Check sheet for the modelled part. Datum: model origin and axes. Units: mm. A direction names the side the tool comes from. Round coordinates to 2 decimals unless told otherwise and drop trailing zeros. Write each loop counter-clockwise with the first axis right and the second up, starting at its lowest first coordinate (ties: lowest second). Pieces come first, ordered by that corner, then holes. Notation, with made-up numbers: M -25.75,79.5 L -7.75,79.5 A26 cw -7.75,97.5 Z; hole C -14.5,66.5 d7. An arc over 180 degrees is marked long. Answer in a Markdown table with one row per item.
```python
from build123d import *

# Parameters (mm, degrees)
SKETCH_1_R       = 1.6
EXTRUDE_1_DEPTH  = 2
CHAMFER_1_SIZE   = 5
FILLET_START     = -1
FILLET_1_DEPTH   = 4
FILLET_1_2_DEPTH = 2
FILLET_2_R       = 3


with BuildPart() as part:
    # 草图1 → 凸台-拉伸1 (new body)
    with BuildSketch(Plane(origin=(0, 0, 0), x_dir=(1, 0, 0), z_dir=(0, 1, 0))):
        Polygon((-10, -14), (-10, 14), (10, 14), (10, 6), (30, 6), (30, -6), (10, -6), (10, -14), align=None)
        with Locations(Location((0, 10, 0), (0, 0, 270))):
            Circle(SKETCH_1_R, mode=Mode.SUBTRACT)
        with Locations(Location((0, -10, 0), (0, 0, 90))):
            Circle(SKETCH_1_R, mode=Mode.SUBTRACT)
        with Locations(Location((17.5, 0, 0), (0, 0, 270))):
            Circle(SKETCH_1_R, mode=Mode.SUBTRACT)
        with Locations(Location((24.5, 0, 0), (0, 0, 270))):
            Circle(SKETCH_1_R, mode=Mode.SUBTRACT)
    extrude(amount=EXTRUDE_1_DEPTH)

    # 倒角1
    chamfer_1_edges = [part.edges().sort_by_distance(p)[0] for p in [
        (10, 1, 14),
        (-10, 1, 14),
        (-10, 1, -14),
        (10, 1, -14),
    ]]
    chamfer(chamfer_1_edges, length=CHAMFER_1_SIZE)

    # 圆角1: read off the stored shape, not the designer's step
    # 圆角1 outline → 圆角1 (cut)
    with BuildSketch(Plane(origin=(0, 0, 0), x_dir=(1, 0, 0), z_dir=(0, 1, 0)).offset(FILLET_START)):
        with BuildLine():
            ThreePointArc((27, 6), (29.121320344, 5.121320344), (30, 3))
            Line((30, 3), (30, 6))
            Line((30, 6), (27, 6))
        make_face()
        with BuildLine():
            ThreePointArc((30, -3), (29.121320344, -5.121320344), (27, -6))
            Line((27, -6), (30, -6))
            Line((30, -6), (30, -3))
        make_face()
    extrude(amount=FILLET_1_DEPTH, mode=Mode.SUBTRACT)

    # Fillet 1 2 outline → Fillet 1 2 (add)
    with BuildSketch(Plane(origin=(0, 0, 0), x_dir=(1, 0, 0), z_dir=(0, 1, 0))):
        with BuildLine():
            Line((10, 6), (13, 6))
            ThreePointArc((13, 6), (10.878679656, 6.878679656), (10, 9))
            Line((10, 9), (10, 6))
        make_face()
        with BuildLine():
            ThreePointArc((10, -9), (10.878679656, -6.878679656), (13, -6))
            Line((13, -6), (10, -6))
            Line((10, -6), (10, -9))
        make_face()
    extrude(amount=FILLET_1_2_DEPTH)

    # 圆角2
    fillet_2_edges = [part.edges().sort_by_distance(p)[0] for p in [
        (10, 1, 9),
        (10, 1, -9),
    ]]
    fillet(fillet_2_edges, radius=FILLET_2_R)


solid = part.part
```
1. Section check A-A, the plane y = 0.85. Record the cut outline in (x, z), and give its area (3 significant figures).
Found:
| item | result |
|---|---|
| outline | M -10,-9 L -5,-14 L 5,-14 L 9.29,-9.71 A3 ccw 10.08,-8.29 A3 cw 13,-6 L 27,-6 A3 ccw 30,-3 L 30,3 A3 ccw 27,6 L 13,6 A3 cw 10.08,8.29 A3 ccw 9.29,9.71 L 5,14 L -5,14 L -10,9 Z; hole C 0,-10 d3.2; hole C 0,10 d3.2; hole C 17.5,0 d3.2; hole C 24.5,0 d3.2 |
| area | 718 mm2 |
2. Section check C-C, the plane x = 24.5. Record the cut outline in (y, z).
Found:
| item | result |
|---|---|
| outline | M 0,-6 L 2,-6 L 2,-1.6 L 0,-1.6 Z; M 0,1.6 L 2,1.6 L 2,6 L 0,6 Z |
3. Go/stop test with flat-tipped pins: pin 1 (5 mm diameter, centred on x = 0, z = 10, fed in from +Y); pin 2 (1.9 mm diameter, centred on x = 17.5, z = 0, fed in from +Y). Record where each tip stops, or that it passes through.
Found:
| item | result |
|---|---|
| pin 1 | stops at y = 2 |
| pin 2 | passes through |
4. Section check B-B, the plane z = 0. Record the cut outline in (x, y).
Found:
| item | result |
|---|---|
| outline | M -10,0 L 15.9,0 L 15.9,2 L -10,2 Z; M 19.1,0 L 22.9,0 L 22.9,2 L 19.1,2 Z; M 26.1,0 L 30,0 L 30,2 L 26.1,2 Z |
5. Section check D-D, the plane x = 0. Record the cut outline in (y, z).
Found:
| item | result |
|---|---|
| outline | M 0,-14 L 2,-14 L 2,-11.6 L 0,-11.6 Z; M 0,-8.4 L 2,-8.4 L 2,8.4 L 0,8.4 Z; M 0,11.6 L 2,11.6 L 2,14 L 0,14 Z |
6. Draft check along Z on faces 4 (the face through (-7, 1, 12)), 5 (the face through (0.07, 0.99, -11.6)), 6 (the face through (29.1, 0.99, -5.14)). Enter one of: +Z half, -Z half, draft (parallel to the pull), parting line (faces both ways), or undercut.
Found:
| item | result |
|---|---|
| face 4 | +Z half |
| face 5 | undercut |
| face 6 | -Z half |
7. Access from +Z, -Z, +X, -X, +Y, -Y to the whole of each face (thin tool, end or side, straight path). Record for faces 1 (the face through (20, 1, -6)), 2 (the face through (0, 1, 14)), 3 (the face through (20, 1, 6)).
Found:
| item | result |
|---|---|
| face 1 | -Z, +X, +Y, -Y |
| face 2 | +Z, +X, -X, +Y, -Y |
| face 3 | +Z, +X, +Y, -Y |
8. Scan lines: L1, parallel to X at y = 1.05, z = 0; L2, parallel to X at y = 0.8, z = 10; L3, parallel to Z at x = 16.5, y = 1.75. Record each from-to range of solid material in increasing order.
Found:
| item | result |
|---|---|
| L1 | x = -10 to 15.9, 19.1 to 22.9, 26.1 to 30 |
| L2 | x = -9 to -1.6, 1.6 to 9 |
| L3 | z = -6 to -1.25, 1.25 to 6 |
